```python
from build123d import *

# Parameters (mm, degrees)
F0_W     = 49.53
F0_H     = 81.28
F1_DEPTH = 6.35
F2_W     = 12.192
F2_H     = 4.572
F3_DEPTH = 2.032
F4_W     = 18.669
F4_H     = 1.016
F5_DEPTH = 0.508


with BuildPart() as f1:
    # F0 (on Top) → F1 (new body)
    with BuildSketch(Plane.XY):
        with Locations((24.765, 40.64)):
            Rectangle(F0_W, F0_H)
    extrude(amount=F1_DEPTH)

    # F2 (on face) → F3 (cut)
    with BuildSketch(Plane.XY.offset(6.35)):
        with Locations((24.765, 6.35)):
            Rectangle(F2_W, F2_H)
        with Locations((24.765, 13.97)):
            Rectangle(F2_W, F2_H)
        with Locations((24.765, 21.59)):
            Rectangle(F2_W, F2_H)
        with Locations((24.765, 29.21)):
            Rectangle(F2_W, F2_H)
        with Locations((24.765, 36.83)):
            Rectangle(F2_W, F2_H)
        with Locations((24.765, 44.45)):
            Rectangle(F2_W, F2_H)
        with Locations((24.765, 52.07)):
            Rectangle(F2_W, F2_H)
        with Locations((24.765, 59.69)):
            Rectangle(F2_W, F2_H)
        with Locations((24.765, 67.31)):
            Rectangle(F2_W, F2_H)
        with Locations((24.765, 74.93)):
            Rectangle(F2_W, F2_H)
    extrude(amount=-F3_DEPTH, mode=Mode.SUBTRACT)

    # F4 (on face) → F5 (join)
    with BuildSketch(Plane.XY.offset(6.35)):
        with Locations((40.1955, 6.35)):
            Rectangle(F4_W, F4_H)
        with Locations((9.3345, 6.35)):
            Rectangle(F4_W, F4_H)
        with Locations((9.3345, 13.97)):
            Rectangle(F4_W, F4_H)
        with Locations((40.1955, 13.97)):
            Rectangle(F4_W, F4_H)
        with Locations((9.3345, 21.59)):
            Rectangle(F4_W, F4_H)
        with Locations((40.1955, 21.59)):
            Rectangle(F4_W, F4_H)
        with Locations((9.3345, 29.21)):
            Rectangle(F4_W, F4_H)
        with Locations((40.1955, 29.21)):
            Rectangle(F4_W, F4_H)
        with Locations((9.3345, 36.83)):
            Rectangle(F4_W, F4_H)
        with Locations((40.1955, 36.83)):
            Rectangle(F4_W, F4_H)
        with Locations((9.3345, 44.45)):
            Rectangle(F4_W, F4_H)
        with Locations((40.1955, 44.45)):
            Rectangle(F4_W, F4_H)
        with Locations((9.3345, 52.07)):
            Rectangle(F4_W, F4_H)
        with Locations((40.1955, 52.07)):
            Rectangle(F4_W, F4_H)
        with Locations((9.3345, 59.69)):
            Rectangle(F4_W, F4_H)
        with Locations((40.1955, 59.69)):
            Rectangle(F4_W, F4_H)
        with Locations((9.3345, 67.31)):
            Rectangle(F4_W, F4_H)
        with Locations((40.1955, 67.31)):
            Rectangle(F4_W, F4_H)
        with Locations((9.3345, 74.93)):
            Rectangle(F4_W, F4_H)
        with Locations((40.1955, 74.93)):
            Rectangle(F4_W, F4_H)
    extrude(amount=F5_DEPTH)


solid = f1.part
```
Source: CAD feature listing. Evaluate the final solid. Frame: model axes, mm. Round coordinates to 2 decimals unless told otherwise and drop trailing zeros. Loops run counter-clockwise (first coordinate to the right, second up) from the corner with the lowest first, then second, coordinate; pieces in that order, holes last.
(1) Pull-direction query (X, two-part tool) for faces 1 (the flat face through (24, 81.28, 3)), 2 (the flat face through (25, 26.924, 5)); classes: +X half, -X half, draft (parallel to the pull), parting line (faces both ways), or undercut.
From the geometry:
face 1: draft
face 2: undercut
(2) Section query B-B (y = 49). Output: boundary loops of the cut face in (x, z).
From the geometry:
outline: (0, 0) - (49.53, 0) - (49.53, 6.35) - (0, 6.35) - close
(3) Material intervals for probe 1 along X at (y, z) = (37, 5.5); probe 2 along Z at (x, y) = (30.5, 57), sorted ascending.
From the geometry:
probe 1: x = 0 to 18.67, 30.86 to 49.53
probe 2: z = 0 to 6.35
(4) Contact query for flat-ended pins moving along their axis: pin 1 Ø3.5 at (x, y) = (23.5, 52.5) entering from +Z; pin 2 Ø5 at (x, y) = (24.5, 74) entering from +Z. Output: stop coordinate, or through.
From the geometry:
pin 1: stops at z = 4.32
pin 2: stops at z = 6.35
(5) Section query A-A (y = 66). Output: boundary loops of the cut face in (x, z), and give its area (3 significant figures).
From the geometry:
outline: (0, 0) - (49.53, 0) - (49.53, 6.35) - (30.86, 6.35) - (30.86, 4.32) - (18.67, 4.32) - (18.67, 6.35) - (0, 6.35) - close
area: 290 mm2
